Design review of the part built by this model. Coordinates are the model's own, in mm. Face numbers are marked on the shaded views. Give positions to 0.01 mm unless a question says otherwise; leave off trailing zeros. Order: outer loops, then holes, each group sorted by start corner. A loop starts at its lowest first (then second) coordinate and runs counter-clockwise, first axis right, second up.
```python
from build123d import *

# Parameters (mm, degrees)
BOSS_EXTRUDE1_DEPTH = 30
SKETCH2_R           = 8.5
CUT_EXTRUDE1_DEPTH  = 52.5
LPATTERN1_COUNT     = 2
LPATTERN1_PITCH     = 150
SKETCH3_R           = 4.75
CUT_EXTRUDE2_DEPTH  = 15
LPATTERN2_COUNT     = 2
LPATTERN2_PITCH     = 83


with BuildPart() as part:
    # Sketch1 → Boss-Extrude1 (new body)
    with BuildSketch(Plane.XY):
        with BuildLine():
            Line((0, 122.5), (0, 180))
            Line((0, 180), (51.5, 180))
            Line((51.5, 180), (51.5, 0))
            Line((51.5, 0), (0, 0))
            Line((0, 0), (0, 57.5))
            ThreePointArc((0, 57.5), (32.5, 90), (0, 122.5))
        make_face()
    extrude(amount=BOSS_EXTRUDE1_DEPTH)

    # Sketch2 → Cut-Extrude1 (cut, through all)
    with BuildSketch(Plane.ZY):
        with Locations((15, 15)):
            Circle(SKETCH2_R)
    cut_extrude1 = extrude(amount=-CUT_EXTRUDE1_DEPTH, mode=Mode.SUBTRACT)

    # LPattern1: Cut-Extrude1 ×2
    with Locations(*[(0, i * LPATTERN1_PITCH, 0) for i in range(1, LPATTERN1_COUNT)]):
        add(cut_extrude1, mode=Mode.SUBTRACT)

    # Sketch3 → Cut-Extrude2 (cut)
    with BuildSketch(Plane.ZY):
        with Locations((15, 48.5)):
            Circle(SKETCH3_R)
    cut_extrude2 = extrude(amount=-CUT_EXTRUDE2_DEPTH, mode=Mode.SUBTRACT)

    # LPattern2: Cut-Extrude2 ×2
    with Locations(*[(0, i * LPATTERN2_PITCH, 0) for i in range(1, LPATTERN2_COUNT)]):
        add(cut_extrude2, mode=Mode.SUBTRACT)


solid = part.part
```
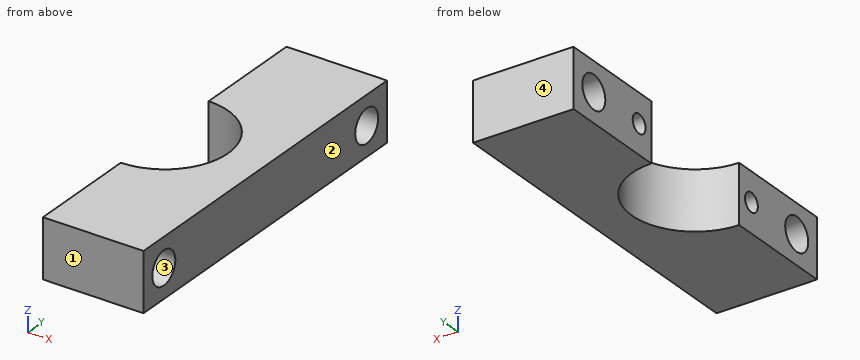
1. Draft analysis for pull direction Y (two halves, no side actions). For the marked faces 1, 2, 3 and 4, state which applies: pulls with the +Y half, pulls with the -Y half, needs draft (parallel to the pull), parting line crosses it, or undercut.
Recorded:
face 1: pulls with the -Y half
face 2: needs draft
face 3: undercut
face 4: pulls with the +Y half
2. For line 1 along Y through (x, z) = (10.75, 15); line 2 along Y through (x, z) = (29, 15); line 3 along Y through (x, z) = (24, 15), list the stretches that pass through material, from the lowest coordinate up.
Recorded:
line 1: y = 0 to 6.5, 23.5 to 43.75, 53.25 to 59.33, 120.67 to 126.75, 136.25 to 156.5, 173.5 to 180
line 2: y = 0 to 6.5, 23.5 to 75.33, 104.67 to 156.5, 173.5 to 180
line 3: y = 0 to 6.5, 23.5 to 68.09, 111.91 to 156.5, 173.5 to 180
3. Take a section at D-D (x = 37). State the section outline as (y, z) points, then the cut area to 3 significant figures.
Recorded:
outline: (0, 0) - (180, 0) - (180, 30) - (0, 30) - close; hole circle Ø17 at (15, 15); hole circle Ø17 at (165, 15)
area: 4,950 mm2
4. For pin 1 (4 mm diameter, centred on y = 110.5, z = 20.5, fed in from -X), flat-tipped, find the tip position at first contact; note if it passes through.
Recorded:
pin 1: stops at x = 23.45
5. Take a section at C-C (z = 13). State the section outline as (x, y) points, then the cut area to 3 significant figures.
Recorded:
outline: (0, 0) - (51.5, 0) - (51.5, 6.74) - (0, 6.74) - close; (0, 23.26) - (51.5, 23.26) - (51.5, 156.74) - (0, 156.74) - (0, 135.81) - (15, 135.81) - (15, 127.19) - (0, 127.19) - (0, 122.5) arc R32.5 cw to (0, 57.5) - (0, 52.81) - (15, 52.81) - (15, 44.19) - (0, 44.19) - close; (0, 173.26) - (51.5, 173.26) - (51.5, 180) - (0, 180) - close
area: 5,650 mm2
6. Take a section at A-A (x = 26). State the section outline as (y, z) points.
Recorded:
outline: (0, 0) - (70.5, 0) - (70.5, 30) - (0, 30) - close; (109.5, 0) - (180, 0) - (180, 30) - (109.5, 30) - close; hole circle Ø17 at (15, 15); hole circle Ø17 at (165, 15)
7. Take a section at B-B (y = 15). State the section outline as (x, z) points, then the cut area to 4 significant figures.
Recorded:
outline: (0, 0) - (51.5, 0) - (51.5, 6.5) - (0, 6.5) - close; (0, 23.5) - (51.5, 23.5) - (51.5, 30) - (0, 30) - close
area: 669.5 mm2
